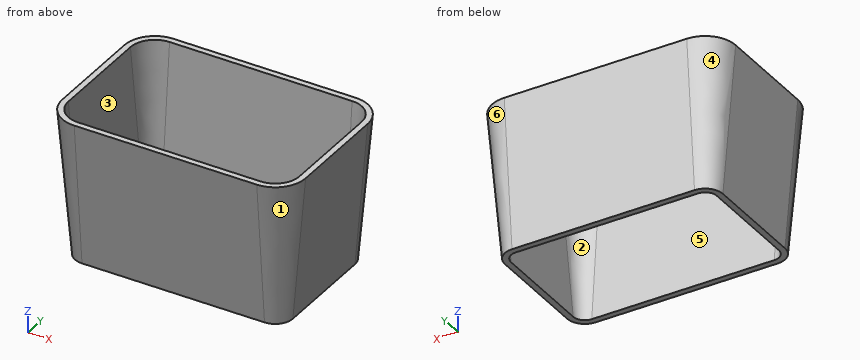
from build123d import *


with BuildPart() as f2:
    # F2: sweep along a path in F0
    with BuildLine(Plane.XY) as f2_path:
        Line((-47.5, 21), (-47.5, -21))
        ThreePointArc((-47.5, -21), (-44.571068, -28.071068), (-37.5, -31))
        Line((-37.5, -31), (37.5, -31))
        ThreePointArc((37.5, -31), (44.571068, -28.071068), (47.5, -21))
        Line((47.5, -21), (47.5, 21))
        ThreePointArc((47.5, 21), (44.571068, 28.071068), (37.5, 31))
        Line((37.5, 31), (-37.5, 31))
        ThreePointArc((-37.5, 31), (-44.571068, 28.071068), (-47.5, 21))
    # F1 (on Front) → F2 (sweep)
    with BuildSketch(Plane.XZ):
        Polygon((-44.75068, -60), (-42.25068, -60), (-47.5, 0), (-50, 0), align=None)
    sweep(path=f2_path.line)


solid = f2.part
Design review of the part built by this model. Coordinates are the model's own, in mm. Face numbers are marked on the shaded views. A direction names the side the tool comes from. Coordinates: 2 decimals unless noted, no trailing zeros. Write each loop counter-clockwise with the first axis right and the second up, starting at its lowest first coordinate (ties: lowest second). Pieces come first, ordered by that corner, then holes. Notation, with made-up numbers: (29, 30.25) -> (81, 30.25) arc R27 ccw to (81, 59.25) -> close; hole circle Ø6 at (63, -28.75). An arc over 180 degrees is marked (long way). Write each question's results on one line, items separated by ' | '. Start each with the question number.
(1) Tool access review of the marked faces 5 and 6: name each direction out of +Z, -Z, +X, -X, +Y, -Y from which nothing blocks a thin tool from reaching the whole face with its end or side.
(2) The part is to be moulded in two halves that separate along Y. For the marked faces 1, 2, 3 and 4, say which applies: pulls with the +Y half, pulls with the -Y half, needs draft (parallel to the pull), parting line crosses it, or undercut.
(3) For line 1 along Y through (x, z) = (-36.5, -32.5); line 2 along X through (y, z) = (25.5, -22); line 3 along Y through (x, z) = (-31.5, -19), list the stretches that pass through material, from the lowest coordinate up. Write a range as from..to.
(4) Take a section at D-D on z = -46. Write out the cut boundary in (x, y).
(5) Take a section at A-A on y = 4.5. Write out the cut boundary in (x, z), and give its area (3 significant figures).
(6) Take a section at C-C on x = 26.5. Write out the cut boundary in (y, z), and give its area (3 significant figures).
(7) Take a section at B-B on z = -36. Write out the cut boundary in (x, y).
(8) Clearance check with flat-ended pins moving along their axes: P1, Ø4, axis at y = 26, z = -50.5, coming from the -X side; P2, Ø12, axis at x = 13.5, z = -37, coming from the +Y side; P3, Ø10, axis at x = 14, z = -40.5, coming from the +Y side. State where each tip first meets the part, or that it passes through.
Results found:
1) face 5: +Z | face 6: -Z, +X, +Y
2) face 1: pulls with the -Y half | face 2: undercut | face 3: undercut | face 4: pulls with the +Y half
3) line 1: y = -30.66..-28.16, 28.16..30.66 | line 2: x = -47.07..-44.21, 44.21..47.07 | line 3: y = -31.84..-29.34, 29.34..31.84
4) outline: (-45.98, -21) arc R8.48 ccw to (-37.5, -29.48) -> (37.5, -29.48) arc R8.48 ccw to (45.98, -21) -> (45.98, 21) arc R8.48 ccw to (37.5, 29.48) -> (-37.5, 29.48) arc R8.48 ccw to (-45.98, 21) -> close; hole (-43.48, -21) arc R5.98 ccw to (-37.5, -26.98) -> (37.5, -26.98) arc R5.98 ccw to (43.48, -21) -> (43.48, 21) arc R5.98 ccw to (37.5, 26.98) -> (-37.5, 26.98) arc R5.98 ccw to (-43.48, 21) -> close
5) outline: (-50, 0) -> (-44.75, -60) -> (-42.25, -60) -> (-47.5, 0) -> close; (42.25, -60) -> (44.75, -60) -> (50, 0) -> (47.5, 0) -> close | area: 300 mm2
6) outline: (-33.5, 0) -> (-28.25, -60) -> (-25.75, -60) -> (-31, 0) -> close; (25.75, -60) -> (28.25, -60) -> (33.5, 0) -> (31, 0) -> close | area: 300 mm2
7) outline: (-46.85, -21) arc R9.35 ccw to (-37.5, -30.35) -> (37.5, -30.35) arc R9.35 ccw to (46.85, -21) -> (46.85, 21) arc R9.35 ccw to (37.5, 30.35) -> (-37.5, 30.35) arc R9.35 ccw to (-46.85, 21) -> close; hole (-44.35, -21) arc R6.85 ccw to (-37.5, -27.85) -> (37.5, -27.85) arc R6.85 ccw to (44.35, -21) -> (44.35, 21) arc R6.85 ccw to (37.5, 27.85) -> (-37.5, 27.85) arc R6.85 ccw to (-44.35, 21) -> close
8) P1: stops at x = -45.03 | P2: stops at y = 30.79 | P3: stops at y = 30.39
